For this review, take the finished solid that the model builds, in its own axes (mm). A direction names the side the tool comes from. Give positions to 0.01 mm unless a question says otherwise; leave off trailing zeros. Order: outer loops, then holes, each group sorted by start corner. A loop starts at its lowest first (then second) coordinate and runs counter-clockwise, first axis right, second up. Notation, with made-up numbers: (41.25, -35.75) - (45.25, -35.75) arc R10 cw to (45.25, -25.75) - close; hole circle Ø4 at (-22, 49). An arc over 180 degrees is marked (long way). One line per item, written item: value.
```python
from build123d import *

# Parameters (mm, degrees)
F0_W     = 70
F0_H     = 85
F0_R     = 1.5
F0_W_2   = 24.796
F0_H_2   = 8.8934727723
F0_R_2   = 19
F1_DEPTH = 1.5
F2_W     = 70
F2_H     = 85
F3_DEPTH = 50
F4_R     = 1.25
F5_DEPTH = 15
F6_R     = 2.5
F7_DEPTH = 3
F8_R     = 0.75
F9_DEPTH = 2.4
F10_R    = 2.4
F11_F1_R = 1.2
F11_F2_R = 1.2


with BuildPart() as f1:
    # F0 (on Top) → F1 (new body)
    with BuildSketch(Plane.XY):
        with Locations((0, -7.5)):
            Rectangle(F0_W, F0_H)
        with Locations((-16.6170093579, -16.6170093579)):
            Circle(F0_R, mode=Mode.SUBTRACT)
        with Locations((0, -33.3067363862)):
            Rectangle(F0_W_2, F0_H_2, mode=Mode.SUBTRACT)
        with Locations((16.6170093579, -16.6170093579)):
            Circle(F0_R, mode=Mode.SUBTRACT)
        with Locations((-16.6170093579, 16.6170093579)):
            Circle(F0_R, mode=Mode.SUBTRACT)
        Circle(F0_R_2, mode=Mode.SUBTRACT)
        with Locations((16.6170093579, 16.6170093579)):
            Circle(F0_R, mode=Mode.SUBTRACT)
    extrude(amount=F1_DEPTH)

    # F2 (on face) → F3 (join)
    with BuildSketch(Plane.XY.offset(1.5)):
        with Locations((0, -7.5)):
            Rectangle(F2_W, F2_H)
        Polygon((-30, 30), (-30, 33.5), (30, 33.5), (30, 30), (33.5, 30), (33.5, -45), (30, -45), (30, -48.5), (-30, -48.5), (-30, -45), (-33.5, -45), (-33.5, 30), align=None, mode=Mode.SUBTRACT)
    extrude(amount=F3_DEPTH)

    # F4 (on face) → F5 (cut)
    with BuildSketch(Plane.XY.offset(51.5)):
        with Locations((-32.5, 32.5)):
            Circle(F4_R)
        with Locations((32.5, -47.5)):
            Circle(F4_R)
        with Locations((32.5, 32.5)):
            Circle(F4_R)
        with Locations((-32.5, -47.5)):
            Circle(F4_R)
    extrude(amount=-F5_DEPTH, mode=Mode.SUBTRACT)

    # F6 (on face) → F7 (join)
    with BuildSketch(Plane.XY):
        with Locations((-16.5714677423, -23.966986686)):
            Circle(F6_R)
        with Locations((12.4001037329, -23.9952448756)):
            Circle(F6_R)
        with Locations((12.3935937881, -44.0698005259)):
            Circle(F6_R)
        with Locations((-16.5627133101, -44.0643951297)):
            Circle(F6_R)
    extrude(amount=F7_DEPTH)

    # F8 (on face) → F9 (cut)
    with BuildSketch(Plane.XY.offset(3)):
        with Locations((-16.5714677423, -23.966986686)):
            Circle(F8_R)
        with Locations((12.4562103301, -23.9926725626)):
            Circle(F8_R)
        with Locations((12.4562103301, -44.1322289407)):
            Circle(F8_R)
        with Locations((-16.5714677423, -44.1322289407)):
            Circle(F8_R)
    extrude(amount=-F9_DEPTH, mode=Mode.SUBTRACT)

    # F10
    f10_edges = [f1.edges().sort_by_distance(p)[0] for p in [
        (-35, 35, 25.75),
        (-35, -50, 25.75),
        (-35, -7.5, 0),
        (0, 35, 0),
        (35, -7.5, 0),
        (0, -50, 0),
        (35, 35, 25.75),
        (35, -50, 25.75),
    ]]
    fillet(f10_edges, radius=F10_R)

    # F11: fillet of radius 1.2 on 23 edges, made by hand

    # F11_f1
    f11_f1_edges = [f1.edges().sort_by_distance(p)[0] for p in [
        (-30, 30, 26.5),
        (30, 30, 26.5),
        (-30, -45, 26.5),
        (30, -45, 26.5),
    ]]
    fillet(f11_f1_edges, radius=F11_F1_R)

    # F11_f2
    f11_f2_edges = [f1.edges().sort_by_distance(p)[0] for p in [
        (0, 33.5, 1.5),
        (-30, 32.35, 1.5),
        (-32.35, 30, 1.5),
        (-30, 33.5, 26.5),
        (-33.5, 30, 26.5),
        (-33.5, -7.5, 1.5),
        (30, 32.35, 1.5),
        (32.35, 30, 1.5),
        (30, 33.5, 26.5),
        (33.5, 30, 26.5),
        (33.5, -7.5, 1.5),
        (-33.5, -45, 26.5),
        (-32.35, -45, 1.5),
        (-30, -48.5, 26.5),
        (0, -48.5, 1.5),
        (30, -47.35, 1.5),
        (32.35, -45, 1.5),
        (33.5, -45, 26.5),
        (30, -48.5, 26.5),
        (30.3514718626, -45.3514718626, 1.5),
        (-30.3514718626, -45.3514718626, 1.5),
        (30.3514718626, 30.3514718626, 1.5),
        (-30.3514718626, 30.3514718626, 1.5),
    ]]
    fillet(f11_f2_edges, radius=F11_F2_R)


solid = f1.part
```
(1) Draft analysis for pull direction Y (two halves, no side actions). For faces 3 (the face through (17.423, 17.882, 0.74)), 4 (the face through (0.456, -49.278, 0.684)), 5 (the face through (0, 34, 51.5)), state which applies: pulls with the +Y half, pulls with the -Y half, needs draft (parallel to the pull), parting line crosses it, or undercut.
Answers below:
face 3: undercut
face 4: pulls with the -Y half
face 5: needs draft
(2) Machinability: for faces 1 (the face through (-34.316, -49.278, 27.294)), 2 (the face through (33.5, -7, 27)), which of the approach directions +Z, -Z, +X, -X, +Y, -Y give a long, thin tool a straight path to every point of the face, cutting with its end or side? Answer none if there is none.
Answers below:
face 1: +Z, -Z, -X, -Y
face 2: +Z
(3) Wall thickness on line 1 (Y direction, x = -32.5, z = 43.5); line 2 (X direction, y = -38.5, z = 23.5); line 3 (Y direction, x = -1, z = 9.5): over which ranges is each line inside the solid? List them lowest first. Write a range as from..to.
Answers below:
line 1: y = -50..-48.75, -46.25..-44.98, 29.98..31.25, 33.75..35
line 2: x = -35..-33.5, 33.5..35
line 3: y = -50..-48.5, 33.5..35
(4) For P1, Ø1.5, axis at x = 12, y = -23, coming from the +Z side; P2, Ø1.5, axis at x = -32.5, y = 32.5, coming from the +Z side; P3, Ø0.9, axis at x = -16.57, y = -23.97, coming from the +Z side, all flat-tipped, find the tip position at first contact; note any pin that passes through.
Answers below:
P1: stops at z = 3
P2: stops at z = 36.5
P3: stops at z = 0.6
(5) Take a section at D-D (y = 26). Write out the cut boundary in (x, z).
Answers below:
outline: (-35, 2.4) arc R2.4 ccw to (-32.6, 0) - (32.6, 0) arc R2.4 ccw to (35, 2.4) - (35, 51.5) - (33.5, 51.5) - (33.5, 2.7) arc R1.2 cw to (32.3, 1.5) - (-32.3, 1.5) arc R1.2 cw to (-33.5, 2.7) - (-33.5, 51.5) - (-35, 51.5) - close
(6) Take a section at B-B (y = 0). Write out the cut boundary in (x, z).
Answers below:
outline: (-35, 2.4) arc R2.4 ccw to (-32.6, 0) - (-19, 0) - (-19, 1.5) - (-32.3, 1.5) arc R1.2 cw to (-33.5, 2.7) - (-33.5, 51.5) - (-35, 51.5) - close; (19, 0) - (32.6, 0) arc R2.4 ccw to (35, 2.4) - (35, 51.5) - (33.5, 51.5) - (33.5, 2.7) arc R1.2 cw to (32.3, 1.5) - (19, 1.5) - close
(7) Take a section at A-A (x = 0). Write out the cut boundary in (y, z), then the cut area to 3 significant figures.
Answers below:
outline: (-50, 2.4) arc R2.4 ccw to (-47.6, 0) - (-37.75, 0) - (-37.75, 1.5) - (-47.3, 1.5) arc R1.2 cw to (-48.5, 2.7) - (-48.5, 51.5) - (-50, 51.5) - close; (-28.86, 0) - (-19, 0) - (-19, 1.5) - (-28.86, 1.5) - close; (19, 0) - (32.6, 0) arc R2.4 ccw to (35, 2.4) - (35, 51.5) - (33.5, 51.5) - (33.5, 2.7) arc R1.2 cw to (32.3, 1.5) - (19, 1.5) - close
area: 205 mm^2
